Geometry: final body of the model. Coordinates: model frame, mm. A direction names the side the tool comes from. Coordinates: 2 decimals unless noted, no trailing zeros. Order: outer loops, then holes, each group sorted by start corner. A loop starts at its lowest first (then second) coordinate and runs counter-clockwise, first axis right, second up. Notation, with made-up numbers: (14.25, 39) - (59.25, 39) arc R20 cw to (59.25, 69) - close; hole circle Ø5 at (28.5, 34). An arc over 180 degrees is marked (long way). Use a Markdown table: item, result. Add a question column.
```python
from build123d import *

# Parameters (mm, degrees)
BOSS_EXTRUDE1_DEPTH     = 30
CUT_EXTRUDE1_DEPTH      = 41.298883359
CUT_EXTRUDE1_DEPTH_BACK = 41.298883359
SKETCH2_R               = 1.65
CUT_EXTRUDE2_DEPTH      = 41.298883359
CUT_EXTRUDE2_DEPTH_BACK = 41.298883359
SKETCH3_R               = 1.65
FILLET1_R               = 5
FILLET2_R               = 3
CHAMFER1_SIZE           = 2
CHAMFER2_SIZE           = 1.5
CUT_EXTRUDE3_DEPTH      = 44
CUT_EXTRUDE3_DEPTH_BACK = 44
FILLET3_R               = 1


with BuildPart() as part:
    # Sketch1 → Boss-Extrude1 (new, symmetric)
    with BuildSketch(Plane(origin=(0, 0, 0), x_dir=(0, 0, -1), z_dir=(1, 0, 0))):
        Polygon((0, 0), (20, 0), (20, 5), (-5, 5), (-5, -18), (0, -18), align=None)
    extrude(amount=BOSS_EXTRUDE1_DEPTH, both=True)

    # Sketch2 → Cut-Extrude1 (cut, two sides: drawn at the far end of the back side and taken through both)
    with BuildSketch(Plane.XY.offset(-CUT_EXTRUDE1_DEPTH_BACK)):
        with Locations((22.5, -12.5)):
            Circle(SKETCH2_R)
        with Locations(Location((-22.5, -12.5, 0), (0, 0, 270))):
            Circle(SKETCH2_R)
    extrude(amount=CUT_EXTRUDE1_DEPTH + CUT_EXTRUDE1_DEPTH_BACK, mode=Mode.SUBTRACT)

    # Sketch3 → Cut-Extrude2 (cut, two sides: drawn at the far end of the back side and taken through both)
    with BuildSketch(Plane(origin=(0, 0, 0), x_dir=(1, 0, 0), z_dir=(0, 1, 0)).offset(-CUT_EXTRUDE2_DEPTH_BACK)):
        with Locations(Location((7, 7, 0), (0, 0, 270))):
            Circle(SKETCH3_R)
        with Locations(Location((17, 7, 0), (0, 0, 270))):
            Circle(SKETCH3_R)
        with Locations(Location((17, 15, 0), (0, 0, 270))):
            Circle(SKETCH3_R)
        with Locations(Location((7, 15, 0), (0, 0, 270))):
            Circle(SKETCH3_R)
        Polygon((21, 20), (27, 10), (30, 10), (38.233411058, 24.132528873), (36.351497345, 35.273458054), (14.220192082, 36.929542121), (-3.211887252, 31.82230336), (-34.48112888, 29.547116003), (-37.048006924, 19.046251277), (-30, 10), (-3, 10), (3, 20), align=None)
    extrude(amount=CUT_EXTRUDE2_DEPTH + CUT_EXTRUDE2_DEPTH_BACK, mode=Mode.SUBTRACT)

    # Fillet1
    fillet1_edges = [part.edges().sort_by_distance(p)[0] for p in [
        (30, -18, 2.5),
        (-30, 2.5, -10),
        (21, 2.5, -20),
        (3, 2.5, -20),
        (-3, 2.5, -10),
        (-30, -18, 2.5),
    ]]
    fillet(fillet1_edges, radius=FILLET1_R)

    # Fillet2
    fillet2_edges = [part.edges().sort_by_distance(p)[0] for p in [
        (0, 5, 5),
        (0, 0, 0),
    ]]
    fillet(fillet2_edges, radius=FILLET2_R)

    # Chamfer1
    chamfer1_edges = [part.edges().sort_by_distance(p)[0] for p in [
        (7, 0, -8.65),
        (17, 0, -16.65),
        (7, 0, -16.65),
        (17, 0, -8.65),
    ]]
    chamfer(chamfer1_edges, length=CHAMFER1_SIZE)

    # Chamfer2
    chamfer2_edges = [part.edges().sort_by_distance(p)[0] for p in [
        (20.85, -12.5, 5),
        (-22.5, -10.85, 5),
    ]]
    chamfer(chamfer2_edges, length=CHAMFER2_SIZE)

    # Sketch4 → Cut-Extrude3 (cut, two sides: drawn at the far end of the back side and taken through both)
    with BuildSketch(Plane.XY.offset(5).offset(-CUT_EXTRUDE3_DEPTH_BACK)):
        with BuildLine():
            Line((-11, -6), (11, -6))
            ThreePointArc((11, -6), (15, -10), (11, -14))
            Line((11, -14), (-11, -14))
            ThreePointArc((-11, -14), (-15, -10), (-11, -6))
        make_face()
    extrude(amount=CUT_EXTRUDE3_DEPTH + CUT_EXTRUDE3_DEPTH_BACK, mode=Mode.SUBTRACT)

    # Fillet3
    fillet3_edges = [part.edges().sort_by_distance(p)[0] for p in [
        (30, 2.5, -10),
        (27, 2.5, -10),
    ]]
    fillet(fillet3_edges, radius=FILLET3_R)


solid = part.part
```
1) Section A-A (x = -9). Return loops of the section in (y, z), then the cut area to 3 significant figures.
2) Section B-B (z = -15). Return loops of the section in (x, y).
3) Pin query (flat end, axial travel): pin 1 (1.5 mm diameter, centred on x = -14, y = -13.5, fed in from -Z); pin 2 (13.5 mm diameter, centred on x = -14, z = -13, fed in from -Y); pin 3 (2.5 mm diameter, centred on x = -15.5, y = 3.5, fed in from -Z). Return the tip coordinate at first contact, or that it passes through.
4) Section D-D (x = 17). Return loops of the section in (y, z), then the cut area to 3 significant figures.
5) Section C-C (x = 7). Return loops of the section in (y, z), then the cut area to 3 significant figures.
6) Ray query, line 1 along Y through (x, z) = (22.5, 0.95); line 2 along Z through (x, y) = (17, 3.2); line 3 along X through (y, z) = (2.9, -15). Return the intervals inside material, ascending.
7) Draft query along X for faces 6 (the face through (-28, 3, -9)), 7 (the face through (18.115, 3.479, -8.216)), 8 (the face through (0, 0, -9)). Return one class per face: pulls with the +X half, pulls with the -X half, needs draft (parallel to the pull), parting line crosses it, or undercut.
8) Set-up query: faces 1 (the face through (-3.336, 2.535, -10.667)), 2 (the face through (15, -10, 2)), 3 (the face through (0, -16, 0)), 4 (the face through (28, 2, -10)), 5 (the face through (17.496, 3.479, -13.426)). Return all of +Z, -Z, +X, -X, +Y, -Y with unobstructed straight access to the full face (end or side cutting, diameter ignored); none if empty.
Values follow:
| question | item | result |
|---|---|---|
| 1 | outline | (-18, 0) - (-14, 0) - (-14, 5) - (-18, 5) - close; (-6, 0) - (-3, 0) arc R3 cw to (0, -3) - (0, -10) - (5, -10) - (5, 2) arc R3 ccw to (2, 5) - (-6, 5) - close |
| 1 | area | 125 mm² |
| 2 | outline | (0, 0) - (3.35, 0) - (5.35, 2) - (5.35, 5) - (0, 5) - close; (8.65, 2) - (10.65, 0) - (13.35, 0) - (15.35, 2) - (15.35, 5) - (8.65, 5) - close; (18.65, 2) - (20.65, 0) - (24, 0) - (24, 5) - (18.65, 5) - close |
| 3 | pin 1 | stops at z = 0 |
| 3 | pin 2 | stops at y = 0 |
| 3 | pin 3 | stops at z = -10 |
| 4 | outline | (-18, 0) - (-3, 0) arc R3 cw to (0, -3) - (0, -3.35) - (2, -5.35) - (5, -5.35) - (5, 2) arc R3 ccw to (2, 5) - (-18, 5) - close; (0, -20) - (5, -20) - (5, -16.65) - (2, -16.65) - (0, -18.65) - close; (0, -11.35) - (2, -13.35) - (5, -13.35) - (5, -8.65) - (2, -8.65) - (0, -10.65) - close |
| 4 | area | 174 mm² |
| 5 | outline | (-18, 0) - (-14, 0) - (-14, 5) - (-18, 5) - close; (-6, 0) - (-3, 0) arc R3 cw to (0, -3) - (0, -3.35) - (2, -5.35) - (5, -5.35) - (5, 2) arc R3 ccw to (2, 5) - (-6, 5) - close; (0, -20) - (5, -20) - (5, -16.65) - (2, -16.65) - (0, -18.65) - close; (0, -11.35) - (2, -13.35) - (5, -13.35) - (5, -8.65) - (2, -8.65) - (0, -10.65) - close |
| 5 | area | 134 mm² |
| 6 | line 1 | y = -18 to -14.15, -10.85 to 5 |
| 6 | line 2 | z = -20 to -16.65, -13.35 to -8.65, -5.35 to 4.75 |
| 6 | line 3 | x = 0 to 5.35, 8.65 to 15.35, 18.65 to 24 |
| 7 | face 6 | pulls with the -X half |
| 7 | face 7 | undercut |
| 7 | face 8 | needs draft |
| 8 | face 1 | -Z, -X, +Y, -Y |
| 8 | face 2 | +Z, -Z |
| 8 | face 3 | -Z, +X, -X, -Y |
| 8 | face 4 | -Z, +X, +Y, -Y |
| 8 | face 5 | +Y, -Y |
